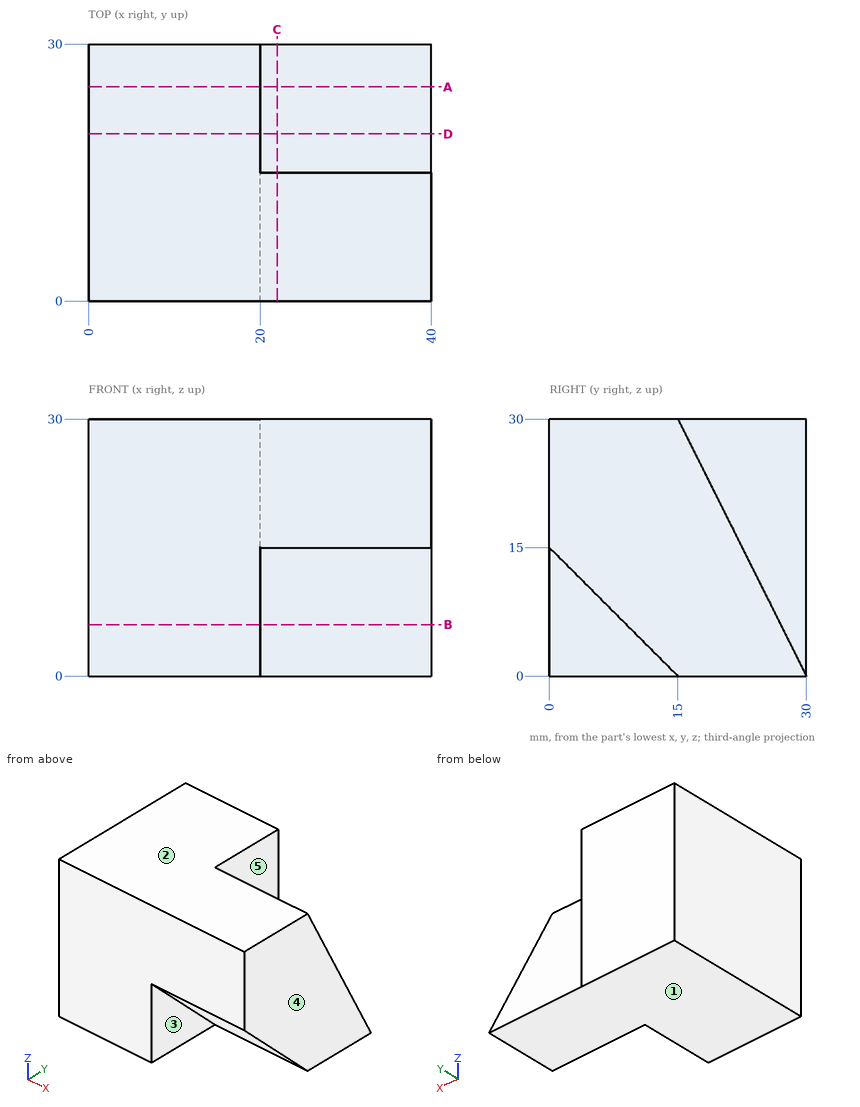
Input: dimensioned drawing with shaded views. Units: mm. Origin: part minimum x, y, z. A direction names the side the tool comes from. Give positions to 0.01 mm unless a question says otherwise; leave off trailing zeros. Write each loop counter-clockwise with the first axis right and the second up, starting at its lowest first coordinate (ties: lowest second). Pieces come first, ordered by that corner, then holes. Notation, with made-up numbers: (-37, -24) - (-17, -24) arc R20 ccw to (-17, -16) - close; hole circle Ø5 at (70.5, 2). An arc over 180 degrees is marked (long way). Write item = value, one per line. Start each with the question number.
1) Cut plane C-C (x = 22). Return loops of the section in (y, z).
2) Cut plane B-B (z = 6). Return loops of the section in (x, y), and give its area (3 significant figures).
3) Reachability of the marked faces 4 and 5 from +Z, -Z, +X, -X, +Y, -Y: full face, straight path, thin tool, end or side. Return the list, or none.
4) Material intervals for L1, parallel to X at y = 27.75, z = 26; L2, parallel to Z at x = 32.5, y = 7.25; L3, parallel to Y at x = 22.5, z = 26.25 (3 decimals), sorted ascending. Write a range as [from, to].
5) Cut plane A-A (y = 25). Return loops of the section in (x, z).
6) Cut plane D-D (y = 19.5). Return loops of the section in (x, z), and give its area (3 significant figures).
7) Pin query (flat end, axial travel): pin 1 (10 mm diameter, centred on x = 32, z = 5.5, fed in from +Y). Return the tip coordinate at first contact, or that it passes through.
8) Draft query along Z for the marked faces 1, 2 and 3. Return one class per face: pulls with the +Z half, pulls with the -Z half, needs draft (parallel to the pull), parting line crosses it, or undercut.
Answers follow:
q1.outline = (0, 15) - (15, 0) - (30, 0) - (15, 30) - (0, 30) - close
q2.outline = (0, 0) - (20, 0) - (20, 9) - (40, 9) - (40, 27) - (20, 27) - (20, 30) - (0, 30) - close
q2.area = 960 mm^2
q3.face_4 = +Z, -Z, +X, +Y, -Y
q3.face_5 = +Z, +X, +Y
q4.L1 = [0, 20]
q4.L2 = [7.75, 30]
q4.L3 = [0, 16.875]
q5.outline = (0, 0) - (40, 0) - (40, 10) - (20, 10) - (20, 30) - (0, 30) - close
q6.outline = (0, 0) - (40, 0) - (40, 21) - (20, 21) - (20, 30) - (0, 30) - close
q6.area = 1,020 mm^2
q7.pin_1 = 29.75
q8.face_1 = pulls with the -Z half
q8.face_2 = pulls with the +Z half
q8.face_3 = needs draft
